Source: three-view drawing plus pictorial views. Frame: mm from the lowest corner of the part. A direction names the side the tool comes from. Round coordinates to 2 decimals unless told otherwise and drop trailing zeros. Loops run counter-clockwise (first coordinate to the right, second up) from the corner with the lowest first, then second, coordinate; pieces in that order, holes last. Notation, with made-up numbers: (-31, -2.5) -> (16, -2.5) arc R8 cw to (16, 8.5) -> close; hole circle Ø11 at (43, 22). An arc over 180 degrees is marked (long way). One line per question, with ' | ' between items. Start each with the question number.
Q1. Mould query, pull axis X, two halves, no side actions, for the marked faces 3, 4, 5 and 6. Classes: pulls with the +X half, pulls with the -X half, needs draft (parallel to the pull), parting line crosses it, or undercut.
Q2. Cut plane C-C on z = 8.5. Return loops of the section in (x, y), and give its area (3 significant figures).
Q3. Access query for the marked faces 1 and 2. Directions: +Z, -Z, +X, -X, +Y, -Y. A direction counts if a zero-diameter tool reaches every point of the face in a straight line with its end or side. Return the directions, or none.
Q4. Cut plane D-D on x = 4. Return loops of the section in (y, z) (3 decimals), and give its area (3 significant figures).
Q5. Contact query for flat-ended pins moving along their axis: P1, Ø1.5, axis at x = 3.5, z = 7, coming from the +Y side; P2, Ø1, axis at x = 6, z = 6.5, coming from the -Y side; P3, Ø4, axis at x = 8.5, y = 7.5, coming from the +Z side; P4, Ø2.5, axis at x = 6.9, y = 6.9, coming from the +Z side. Output: stop coordinate, or through.
Q6. Material intervals for L1, parallel to Y at x = 6.9, z = 3.95; L2, parallel to Y at x = 6.9, z = 8.3, sorted ascending.
Q7. Cut plane A-A on y = 6.9. Return loops of the section in (x, z), and give its area (4 significant figures).
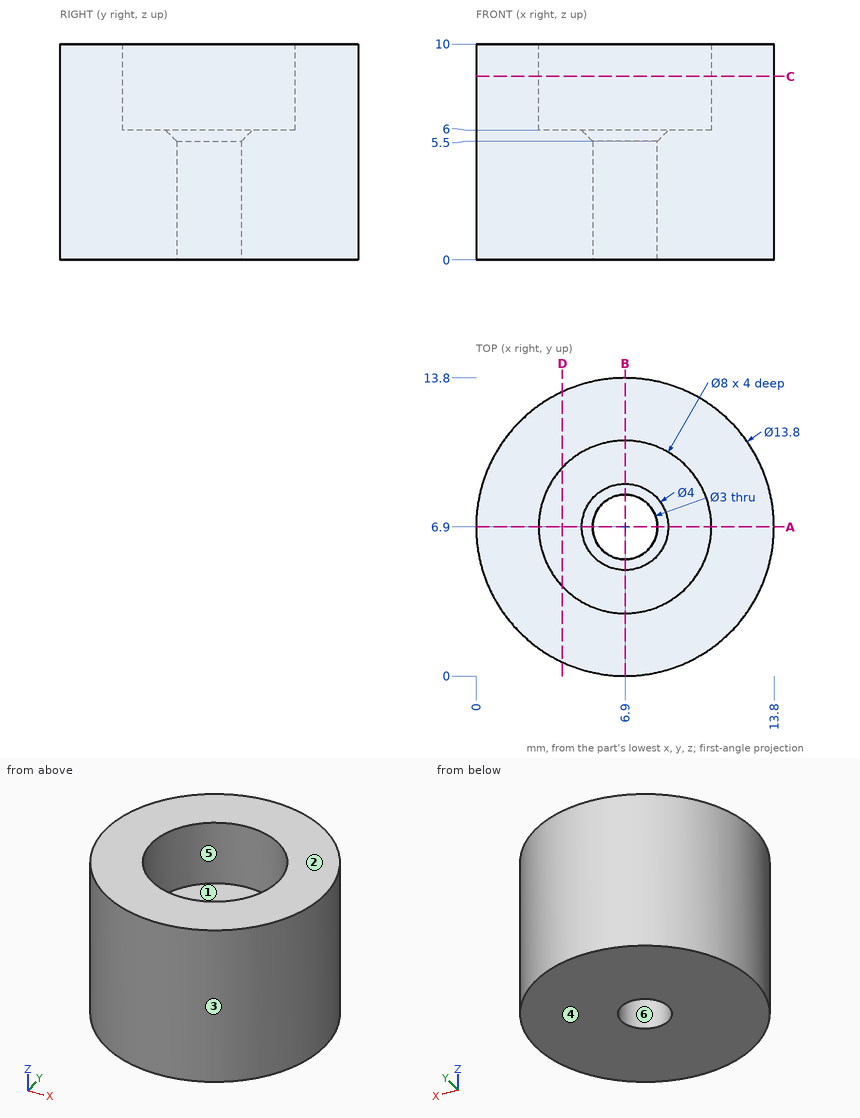
Results:
1) face 3: parting line crosses it | face 4: needs draft | face 5: undercut | face 6: undercut
2) outline: circle Ø13.8 at (6.9, 6.9); hole circle Ø8 at (6.9, 6.9) | area: 99.3 mm^2
3) face 1: +Z | face 2: +Z, +X, -X, +Y, -Y
4) outline: (0.639, 0) -> (13.161, 0) -> (13.161, 10) -> (9.655, 10) -> (9.655, 6) -> (4.145, 6) -> (4.145, 10) -> (0.639, 10) -> close | area: 103 mm^2
5) P1: y = 13.27 | P2: y = 0.01 | P3: z = 6 | P4: through
6) L1: 0 to 5.4, 8.4 to 13.8 | L2: 0 to 2.9, 10.9 to 13.8
7) outline: (0, 0) -> (5.4, 0) -> (5.4, 5.5) -> (4.9, 6) -> (2.9, 6) -> (2.9, 10) -> (0, 10) -> close; (8.4, 0) -> (13.8, 0) -> (13.8, 10) -> (10.9, 10) -> (10.9, 6) -> (8.9, 6) -> (8.4, 5.5) -> close | area: 87.75 mm^2
